Can you work these out from the model? Positions are in its coordinate system, mm. A direction names the side the tool comes from. Round coordinates to 2 decimals unless told otherwise and drop trailing zeros. Write each loop counter-clockwise with the first axis right and the second up, starting at its lowest first coordinate (ties: lowest second). Pieces come first, ordered by that corner, then holes. Notation, with made-up numbers: M -29,-1.5 L 2,-1.5 A26 ccw 2,20.5 Z; hole C 66.5,45 d3. An arc over 180 degrees is marked long. Answer as a JSON object with one key per item and string values. Group by question number.
1) Suppose I cut it at B-B, the plane x = 110.5. Write out the boundary of the cut face in (y, z), and give its area (3 significant figures).
2) If we mould it in two halves opening along X, with no side actions, what happens to faces 1 (the cylindrical face through (58, 15, -59)), 2 (the flat face through (1.5, 10, -32)), 3 (the flat face through (130, 15, -58))? For each: +X half, -X half, draft (parallel to the pull), parting line (faces both ways), or undercut.
3) I'm going to push flat-ended pins straight in: pin 1 Ø3 at (x, z) = (29, -16) entering from +Y; pin 2 Ø3 at (x, z) = (86.5, -58.5) entering from -Y. Where does each tip first touch, or does it pass through?
4) Suppose I cut it at A-A, the plane x = 19. Write out the boundary of the cut face in (y, z), and give its area (3 significant figures).
5) On a 3-axis mill with a long thin cutter (end or side, diameter ignored), from which of +Z, -Z, +X, -X, +Y, -Y can I reach the whole of each face in a straight line? I mean faces 4 (the flat face through (62.039, 2.465, -20.976)), 5 (the flat face through (80, 20, -5)), 6 (the cylindrical face through (27, -3, -43)), 7 (the flat face through (130, 15, -6)). Say none if no direction works.
6) Please list where these lines run through material, in increasing order: L1, parallel to X at y = 15, z = -5; L2, parallel to X at y = -2.9, z = -17; L3, parallel to Y at x = 117, z = -59.25. Write a range as [from, to].
7) Suppose I cut it at C-C, the plane y = 12. State how many separate pieces and enclosed holes the cut face has, and give its area (3 significant figures).
from build123d import *

# Parameters (mm, degrees)
SKETCH_1_W           = 160
SKETCH_1_H           = 64
EXTRUDE_1_DEPTH      = 5
SKETCH_2_W           = 100
SKETCH_2_H           = 7
SKETCH_2_W_2         = 5
SKETCH_2_H_2         = 30
EXTRUDE_2_DEPTH      = 20
FILLET_1_R           = 5
SKETCH_3_R           = 5
SKETCH_3_R_2         = 1.7
EXTRUDE_3_DEPTH      = 5
SKETCH_4_R           = 2.75
CUT_EXTRUDE_1_DEPTH  = 5
SKETCH_5_W           = 160
SKETCH_5_H           = 2
CUT_EXTRUDE_2_DEPTH  = 64
CUT_EXTRUDE_3_DEPTH  = 7
SKETCH_7_W           = 13
SKETCH_7_H           = 17
CUT_EXTRUDE_4_DEPTH  = 7
SKETCH_8_R           = 5
CUT_EXTRUDE_5_DEPTH  = 67
CUT_EXTRUDE_6_DEPTH  = 1
CUT_EXTRUDE_START    = -9
SKETCH_10_W          = 50
SKETCH_10_H          = 3
CUT_EXTRUDE_7_DEPTH  = 24
SKETCH_12_W          = 160
SKETCH_12_H          = 1.5
CUT_EXTRUDE_11_DEPTH = 34
SKETCH_13_W          = 1.5
SKETCH_13_H          = 57
CUT_EXTRUDE_12_DEPTH = 34
FILLET_2_R           = 1


with BuildPart() as part:
    # 草图1 → 凸台-拉伸1 (new body)
    with BuildSketch(Plane(origin=(0, 0, 0), x_dir=(1, 0, 0), z_dir=(0, 1, 0))):
        with Locations((80, 32)):
            Rectangle(SKETCH_1_W, SKETCH_1_H)
    extrude(amount=EXTRUDE_1_DEPTH)

    # 草图2 → 凸台-拉伸2 (add)
    with BuildSketch(Plane(origin=(0, 5, 0), x_dir=(1, 0, 0), z_dir=(0, 1, 0))):
        with Locations((80, 60.5)):
            Rectangle(SKETCH_2_W, SKETCH_2_H)
        with Locations((157.5, 32)):
            Rectangle(SKETCH_2_W_2, SKETCH_2_H_2)
        with Locations((2.5, 32)):
            Rectangle(SKETCH_2_W_2, SKETCH_2_H_2)
        with Locations((80, 3.5)):
            Rectangle(SKETCH_2_W, SKETCH_2_H)
    extrude(amount=EXTRUDE_2_DEPTH)

    # 圆角1
    fillet_1_edges = [part.edges().sort_by_distance(p)[0] for p in [
        (80, 5, -57),
        (155, 5, -32),
        (5, 5, -32),
        (80, 5, -7),
    ]]
    fillet(fillet_1_edges, radius=FILLET_1_R)

    # 草图3 → 凸台-拉伸3 (add)
    # profile 1 of 4: a face of its own
    with BuildSketch(Plane.XZ):
        with Locations(Location((130, -17, 0), (0, 0, 270))):
            Circle(SKETCH_3_R)
        with Locations(Location((130, -17, 0), (0, 0, 270))):
            Circle(SKETCH_3_R_2, mode=Mode.SUBTRACT)
    # profile 2 of 4: a face of its own
    with BuildSketch(Plane.XZ):
        with Locations(Location((130, -47, 0), (0, 0, 270))):
            Circle(SKETCH_3_R)
        with Locations(Location((130, -47, 0), (0, 0, 270))):
            Circle(SKETCH_3_R_2, mode=Mode.SUBTRACT)
    # profile 3 of 4: a face of its own
    with BuildSketch(Plane.XZ):
        with Locations(Location((30, -47, 0), (0, 0, 270))):
            Circle(SKETCH_3_R)
        with Locations(Location((30, -47, 0), (0, 0, 270))):
            Circle(SKETCH_3_R_2, mode=Mode.SUBTRACT)
    # profile 4 of 4: a face of its own
    with BuildSketch(Plane.XZ):
        with Locations(Location((30, -17, 0), (0, 0, 270))):
            Circle(SKETCH_3_R)
        with Locations(Location((30, -17, 0), (0, 0, 270))):
            Circle(SKETCH_3_R_2, mode=Mode.SUBTRACT)
    extrude(amount=EXTRUDE_3_DEPTH)

    # 草图4 → 切除-拉伸1 (cut)
    with BuildSketch(Plane(origin=(0, 5, 0), x_dir=(1, 0, 0), z_dir=(0, 1, 0))):
        with Locations(Location((130, 17, 0), (0, 0, 270))):
            Circle(SKETCH_4_R)
        with Locations(Location((130, 47, 0), (0, 0, 270))):
            Circle(SKETCH_4_R)
        with Locations(Location((30, 17, 0), (0, 0, 270))):
            Circle(SKETCH_4_R)
        with Locations(Location((30, 47, 0), (0, 0, 270))):
            Circle(SKETCH_4_R)
    extrude(amount=-CUT_EXTRUDE_1_DEPTH, mode=Mode.SUBTRACT)

    # 草图5 → 切除-拉伸2 (cut)
    with BuildSketch(Plane(origin=(0, 25, 0), x_dir=(1, 0, 0), z_dir=(0, 1, 0))):
        with Locations((80, 63)):
            Rectangle(SKETCH_5_W, SKETCH_5_H)
        with Locations((80, 1)):
            Rectangle(SKETCH_5_W, SKETCH_5_H)
    extrude(amount=-CUT_EXTRUDE_2_DEPTH, mode=Mode.SUBTRACT)

    # 草图6 → 切除-拉伸3 (cut)
    with BuildSketch(Plane.XZ):
        Polygon((43.567425452, -51), (116.432574548, -51), (80, -35.2677519), align=None)
        Polygon((36, -47.7322481), (36, -16.2677519), (72.432574548, -32), align=None)
        Polygon((43.567425452, -13), (116.432574548, -13), (80, -28.7322481), align=None)
        Polygon((124, -47.7322481), (124, -16.2677519), (87.567425452, -32), align=None)
    extrude(amount=-CUT_EXTRUDE_3_DEPTH, mode=Mode.SUBTRACT)

    # 草图7 → 切除-拉伸4 (cut)
    with BuildSketch(Plane(origin=(0, 5, 0), x_dir=(1, 0, 0), z_dir=(0, 1, 0))):
        with Locations((17.5, 43.5)):
            Rectangle(SKETCH_7_W, SKETCH_7_H)
        with Locations((17.5, 20.5)):
            Rectangle(SKETCH_7_W, SKETCH_7_H)
        with Locations((142.5, 43.5)):
            Rectangle(SKETCH_7_W, SKETCH_7_H)
        with Locations((142.5, 20.5)):
            Rectangle(SKETCH_7_W, SKETCH_7_H)
    extrude(amount=-CUT_EXTRUDE_4_DEPTH, mode=Mode.SUBTRACT)

    # 草图8 → 切除-拉伸5 (cut)
    with BuildSketch(Plane.XY.offset(-2)):
        with Locations((43, 15)):
            Circle(SKETCH_8_R)
        with Locations((117, 15)):
            Circle(SKETCH_8_R)
        with BuildLine():
            Line((63, 20), (97, 20))
            ThreePointArc((97, 20), (102, 15), (97, 10))
            Line((97, 10), (63, 10))
            ThreePointArc((63, 10), (58, 15), (63, 20))
        make_face()
    extrude(amount=-CUT_EXTRUDE_5_DEPTH, mode=Mode.SUBTRACT)

    # 草图9 → 切除-拉伸6 (cut)
    with BuildSketch(Plane(origin=(160, 0, 0), x_dir=(0, 0, -1), z_dir=(1, 0, 0))):
        Polygon((2, 4.416741909), (2.583258091, 5), (2, 5), align=None)
    extrude(amount=-CUT_EXTRUDE_6_DEPTH, mode=Mode.SUBTRACT)

    # 草图10 → 切除-拉伸7 (cut)
    with BuildSketch(Plane(origin=(0, 1.208370955, 1.208370955), x_dir=(1, 0, 0), z_dir=(0, 0.7071067811865486, 0.7071067811865465)).offset(CUT_EXTRUDE_START)):
        with Locations((80, 4.914213562)):
            Rectangle(SKETCH_10_W, SKETCH_10_H)
    cut_extrude_7 = extrude(amount=CUT_EXTRUDE_7_DEPTH, mode=Mode.SUBTRACT)

    # 镜向1: 切除-拉伸7 across plane
    add(cut_extrude_7.mirror(Plane.XY.offset(-32)), mode=Mode.SUBTRACT)

    # 草图12 → 切除-拉伸11 (cut)
    with BuildSketch(Plane.XZ):
        with Locations((80, -2.75)):
            Rectangle(SKETCH_12_W, SKETCH_12_H)
        with Locations((80, -61.25)):
            Rectangle(SKETCH_12_W, SKETCH_12_H)
    extrude(amount=-CUT_EXTRUDE_11_DEPTH, mode=Mode.SUBTRACT)

    # 草图13 → 切除-拉伸12 (cut)
    with BuildSketch(Plane.XZ):
        with Locations((159.25, -32)):
            Rectangle(SKETCH_13_W, SKETCH_13_H)
        with Locations((0.75, -32)):
            Rectangle(SKETCH_13_W, SKETCH_13_H)
    extrude(amount=-CUT_EXTRUDE_12_DEPTH, mode=Mode.SUBTRACT)

    # 圆角2
    fillet_2_edges = [part.edges().sort_by_distance(p)[0] for p in [
        (130, 0, -12),
        (130, 0, -42),
        (30, 0, -42),
        (30, 0, -12),
    ]]
    fillet(fillet_2_edges, radius=FILLET_2_R - 0.0001)  # a hair under: the kernel refuses the full size


solid = part.part
Results:
{
 "1": {"outline": "M 0,-60.5 L 25,-60.5 L 25,-57 L 10,-57 A5 cw 5,-52 L 5,-51 L 0,-51 Z; M 0,-48.44 L 5,-48.44 L 5,-41.9 L 0,-41.9 Z; M 0,-22.1 L 5,-22.1 L 5,-15.56 L 0,-15.56 Z; M 0,-13 L 5,-13 L 5,-12 A5 cw 10,-7 L 25,-7 L 25,-3.5 L 0,-3.5 Z", "area": "311 mm^2"},
 "2": {"face 1": "undercut", "face 2": "-X half", "face 3": "+X half"},
 "3": {"pin 1": "y = 5", "pin 2": "y = 0"},
 "4": {"outline": "M 0,-60.5 L 5,-60.5 L 5,-52 L 0,-52 Z; M 0,-35 L 5,-35 L 5,-29 L 0,-29 Z; M 0,-12 L 5,-12 L 5,-3.5 L 0,-3.5 Z", "area": "115 mm^2"},
 "5": {"face 4": "+Y, -Y", "face 5": "+Z, -Z", "face 6": "-Y", "face 7": "+Z, -Z, +X, +Y"},
 "6": {"L1": "[30, 38], [48, 58], [102, 112], [122, 130]", "L2": "[25, 28.3], [31.7, 35], [125, 128.3], [131.7, 135]", "L3": "[0, 10], [20, 25]"},
 "7": {"separate pieces": "10", "enclosed holes": "0", "area": "504 mm^2"}
}
